Geometry check sheet. Reference: the model listing, model coordinates, mm. A direction names the side the tool comes from. Coordinates: 2 decimals unless noted, no trailing zeros. Write each loop counter-clockwise with the first axis right and the second up, starting at its lowest first coordinate (ties: lowest second). Pieces come first, ordered by that corner, then holes. Notation, with made-up numbers: (24, -27) -> (33, -27) arc R18 cw to (33, -12) -> close; hole circle Ø11 at (4, -13.75). An arc over 180 degrees is marked (long way). One line per question, with ' | ' between items.
```python
from build123d import *

# Parameters (mm, degrees)
EXTRUDE_1_DEPTH     = 3
EXTRUDE_2_DEPTH     = 20
CUT_EXTRUDE_1_DEPTH = 41
CUT_EXTRUDE_2_DEPTH = 16.2


with BuildPart() as part:
    # Sketch 1 → Extrude 1 (new body)
    with BuildSketch(Plane(origin=(0, 0, 0), x_dir=(1, 0, 0), z_dir=(0, 1, 0))):
        Polygon((40, 15.2), (15.2, 15.2), (15.2, 40), (12.2, 40), (12.2, 12.2), (40, 12.2), align=None)
        Polygon((40, 3), (40, 12.2), (12.2, 12.2), (12.2, 40), (3, 40), (3, 3), align=None)
        Polygon((40, 0), (40, 3), (3, 3), (3, 40), (0, 40), (0, 0), align=None)
    extrude(amount=-EXTRUDE_1_DEPTH)

    # Sketch 1_3 → Extrude 2 (add)
    with BuildSketch(Plane(origin=(0, 0, 0), x_dir=(1, 0, 0), z_dir=(0, 1, 0))):
        Polygon((40, 0), (40, 3), (3, 3), (3, 40), (0, 40), (0, 0), align=None)
        Polygon((40, 15.2), (15.2, 15.2), (15.2, 40), (12.2, 40), (12.2, 12.2), (40, 12.2), align=None)
    extrude(amount=EXTRUDE_2_DEPTH)

    # Sketch 2 → Cut-Extrude 1 (cut, through all)
    with BuildSketch(Plane.ZY):
        Polygon((-40, 8.5), (-28.5, 20), (-40, 20), align=None)
    extrude(amount=-CUT_EXTRUDE_1_DEPTH, mode=Mode.SUBTRACT)

    # Sketch 3 → Cut-Extrude 2 (cut, through all)
    with BuildSketch(Plane(origin=(0, 0, -15.2), x_dir=(-1, 0, 0), z_dir=(0, 0, -1))):
        Polygon((-40, 8.5), (-28.5, 20), (-40, 20), align=None)
    extrude(amount=-CUT_EXTRUDE_2_DEPTH, mode=Mode.SUBTRACT)


solid = part.part
```
(1) Cross-section at A-A (y = 16.5). Record the cut outline in (x, z), plus the area to 3 significant figures.
Answers below:
outline: (0, -32) -> (3, -32) -> (3, -3) -> (32, -3) -> (32, 0) -> (0, 0) -> close; (12.2, -32) -> (15.2, -32) -> (15.2, -15.2) -> (32, -15.2) -> (32, -12.2) -> (12.2, -12.2) -> close | area: 293 mm²
(2) Tool access check on faces 4 (the face through (17, 20, -15)), 5 (the face through (28, 9, -15.2)), 6 (the face through (26, 10, -12.2)), 7 (the face through (12.2, 10, -26)). Record the directions out of +Z, -Z, +X, -X, +Y, -Y that give a thin tool (end or side, any length) a straight path to the whole face; none if there is none.
Answers below:
face 4: +Z, -Z, +X, -X, +Y | face 5: -Z, +X, +Y, -Y | face 6: +X, +Y | face 7: -Z, +Y
(3) Cross-section at B-B (z = -24). Record the cut outline in (x, y).
Answers below:
outline: (0, -3) -> (15.2, -3) -> (15.2, 20) -> (12.2, 20) -> (12.2, 0) -> (3, 0) -> (3, 20) -> (0, 20) -> close
(4) Draft check along X on faces 1 (the face through (34.3, 14.2, -13.7)), 2 (the face through (20, 8, 0)), 3 (the face through (13, 0, -9)). Enter one of: pulls with the +X half, pulls with the -X half, needs draft (parallel to the pull), parting line crosses it, or undercut.
Answers below:
face 1: pulls with the +X half | face 2: needs draft | face 3: undercut
(5) Material ranges on line 1 (X direction, y = 8, z = -25); line 2 (Z direction, x = 28.5, y = 1.75); line 3 (Z direction, x = 13, y = 6), recorded low to high.
Answers below:
line 1: x = 0 to 3, 12.2 to 15.2 | line 2: z = -15.2 to -12.2, -3 to 0 | line 3: z = -40 to -12.2, -3 to 0
(6) Cross-section at C-C (x = 37). Record the cut outline in (y, z).
Answers below:
outline: (-3, -15.2) -> (11.5, -15.2) -> (11.5, -12.2) -> (0, -12.2) -> (0, -3) -> (11.5, -3) -> (11.5, 0) -> (-3, 0) -> close
(7) Depth check by flat-ended pin: P1, Ø2, axis at x = 13, y = 10.5, coming from the -Z side; P2, Ø4, axis at x = 31.5, y = 12, coming from the -Z side; P3, Ø6, axis at y = 12.5, z = -17, coming from the +X side. Enter the tip coordinate at first touch or a pass-through.
Answers below:
P1: stops at z = -39 | P2: stops at z = -15.2 | P3: stops at x = 38.4
(8) Cross-section at D-D (y = 1.5). Record the cut outline in (x, z), plus the area to 3 significant figures.
Answers below:
outline: (0, -40) -> (3, -40) -> (3, -3) -> (40, -3) -> (40, 0) -> (0, 0) -> close; (12.2, -40) -> (15.2, -40) -> (15.2, -15.2) -> (40, -15.2) -> (40, -12.2) -> (12.2, -12.2) -> close | area: 389 mm²
